Model file for the job. Use its own axes, mm. Face numbers are marked on the shaded views. A direction names the side the tool comes from. Give positions to 0.01 mm unless a question says otherwise; leave off trailing zeros. Order: outer loops, then holes, each group sorted by start corner. A loop starts at its lowest first (then second) coordinate and runs counter-clockwise, first axis right, second up. Notation, with made-up numbers: M 31.25,15 L 70.25,15 A25 cw 70.25,53 Z; hole C -30,37 d9. An arc over 180 degrees is marked long. Return JSON: item names as keys, results as strings. Group by question number.
1. Slice it at D-D on x = 11. List the corners of the cut face in (y, z).
2. Pin check, flat tips, straight feed: pin 1 (1 mm diameter, centred on y = 56, z = 14, fed in from +X); pin 2 (3 mm diameter, centred on x = 23, y = 19, fed in from -Z); pin 3 (2 mm diameter, centred on x = -27, z = 3.5, fed in from +Y); pin 4 (2 mm diameter, centred on y = 41.5, z = 8.5, fed in from +X). Stop position of each tip, or through.
3. 3-axis set-ups, long thin cutter, end or side, ignore diameter. For the marked faces 1, 2 and 3: which of +Z, -Z, +X, -X, +Y, -Y reach the whole face in a straight line?
4. Slice it at C-C on y = 59. List the corners of the cut face in (x, z), then the cut area to 3 significant figures.
5. Wall check: probe 1 along Y at (x, z) = (23.5, 13); probe 2 along X at (y, z) = (59, 13.75); probe 3 along X at (y, z) = (65.5, 12). Give the ranges that are in metal, low to high. Write a range as [from, to].
6. Slice it at A-A on z = 9.15. Give the number of separate pieces and of enclosed holes in the cut face, then the cut area to 3 significant figures.
7. Two-plate mould, pull along X, no slides. Class the marked faces 4, 5 and 6: released by +X, released by -X, zero draft, split by the parting line, or undercut.
from build123d import *

# Parameters (mm, degrees)
SKETCH_W             = 60
SKETCH_H             = 60
PAD_DEPTH            = 4
SKETCH001_R          = 3.5
SKETCH001_R_2        = 1.25
PAD001_DEPTH         = 8
SKETCH009_W          = 5
SKETCH009_H          = 25
POCKET008_DEPTH      = 4
PAD006_DEPTH         = 4
SKETCH015_W          = 22
SKETCH015_H          = 4
PAD007_DEPTH         = 2
SKETCH003_R          = 2.25
PAD008_DEPTH         = 8
SKETCH014_R          = 3.5
SKETCH014_R_2        = 1.25
PAD009_DEPTH         = 15
POCKET_DEPTH         = 4
BODY_PLACEMENT_ANGLE = 180


with BuildPart() as part:
    # Sketch → Pad (new body)
    with BuildSketch(Plane.XY):
        Rectangle(SKETCH_W, SKETCH_H)
    extrude(amount=PAD_DEPTH)

    # Sketch001 (on Face6 of Pad) → Pad001 (join)
    with BuildSketch(Plane.XY.offset(4)):
        with Locations((-17, 17)):
            Circle(SKETCH001_R)
        with Locations((-17, 17)):
            Circle(SKETCH001_R_2, mode=Mode.SUBTRACT)
        with Locations((-17, -17)):
            Circle(SKETCH001_R)
        with Locations((-17, -17)):
            Circle(SKETCH001_R_2, mode=Mode.SUBTRACT)
        with Locations((17, -17)):
            Circle(SKETCH001_R)
        with Locations((17, -17)):
            Circle(SKETCH001_R_2, mode=Mode.SUBTRACT)
        with Locations((17, 17)):
            Circle(SKETCH001_R)
        with Locations((17, 17)):
            Circle(SKETCH001_R_2, mode=Mode.SUBTRACT)
    extrude(amount=PAD001_DEPTH)

    # Sketch009 → Pocket008 (cut)
    with BuildSketch(Plane(origin=(0, 0, 0), x_dir=(1, 0, 0), z_dir=(0, 0, -1))):
        Rectangle(SKETCH009_W, SKETCH009_H)
        with Locations((10, 0)):
            Rectangle(SKETCH009_W, SKETCH009_H)
        with Locations((20, 0)):
            Rectangle(SKETCH009_W, SKETCH009_H)
        with Locations((-10, 0)):
            Rectangle(SKETCH009_W, SKETCH009_H)
        with Locations((-20, 0)):
            Rectangle(SKETCH009_W, SKETCH009_H)
    extrude(amount=-POCKET008_DEPTH, mode=Mode.SUBTRACT)

    # Sketch012 (on Face5 of Pocket008) → Pad006 (join)
    with BuildSketch(Plane.XY.offset(4)):
        Polygon((-30, -12), (-35, -12), (-35, -30), (-33, -28), (-33, -16), (-30, -16), align=None)
    pad006 = extrude(amount=-PAD006_DEPTH)

    # Mirrored005: Pad006 across Sketch012 V_Axis
    add(pad006.mirror(Plane(origin=(0, 0, 4), x_dir=(0, 0, 1), z_dir=(1, 0, 0))))

    # Sketch015 (on Face4 of Pad) → Pad007 (join)
    with BuildSketch(Plane(origin=(-30, 0, 0), x_dir=(0, -1, 0), z_dir=(-1, 0, 0))):
        with Locations((0, 2)):
            Rectangle(SKETCH015_W, SKETCH015_H)
    pad007 = extrude(amount=PAD007_DEPTH)

    # Sketch003 (on Face42 of Pad007) → Pad008 (join)
    with BuildSketch(Plane(origin=(-32, 0, 0), x_dir=(0, -1, 0), z_dir=(-1, 0, 0))):
        with BuildLine():
            ThreePointArc((11, 19), (0, 25.938622), (-11, 19))
            Line((-11, 19), (-11, 0))
            Line((11, 0), (-11, 0))
            Line((11, 19), (11, 0))
        make_face()
        with Locations((0, 13.75)):
            Circle(SKETCH003_R, mode=Mode.SUBTRACT)
    pad008 = extrude(amount=PAD008_DEPTH)

    # Sketch014 → Pad009 (join)
    with BuildSketch(Plane.XY.offset(4)):
        with Locations((-23.5, 23.5)):
            Circle(SKETCH014_R)
        with Locations((-23.5, 23.5)):
            Circle(SKETCH014_R_2, mode=Mode.SUBTRACT)
        with Locations((23.5, 23.5)):
            Circle(SKETCH014_R)
        with Locations((23.5, 23.5)):
            Circle(SKETCH014_R_2, mode=Mode.SUBTRACT)
        with Locations((23.5, -23.5)):
            Circle(SKETCH014_R)
        with Locations((23.5, -23.5)):
            Circle(SKETCH014_R_2, mode=Mode.SUBTRACT)
        with Locations((-23.5, -23.5)):
            Circle(SKETCH014_R)
        with Locations((-23.5, -23.5)):
            Circle(SKETCH014_R_2, mode=Mode.SUBTRACT)
    extrude(amount=PAD009_DEPTH)

    # Sketch016 (on Face58 of Pad009) → Pocket (cut)
    with BuildSketch(Plane.YZ.offset(-32)):
        Polygon((-3.637307, 15.85), (-3.637307, 11.65), (0, 9.55), (3.637307, 11.65), (3.637307, 15.85), (0, 17.95), align=None)
    pocket = extrude(amount=-POCKET_DEPTH, mode=Mode.SUBTRACT)

    # Mirrored: Pad007, Pad008 across YZ
    add(pad007.mirror(Plane.YZ))
    add(pad008.mirror(Plane.YZ))

    # Mirrored006: Pocket across YZ
    add(pocket.mirror(Plane.YZ), mode=Mode.SUBTRACT)


with BuildPart() as part_1:
    # Body placement: moved
    add(part.part.moved(Location((0, 42, 22.9))).rotate(Axis((0, 42, 22.9), (1, 0, 0)), BODY_PLACEMENT_ANGLE))


solid = part_1.part
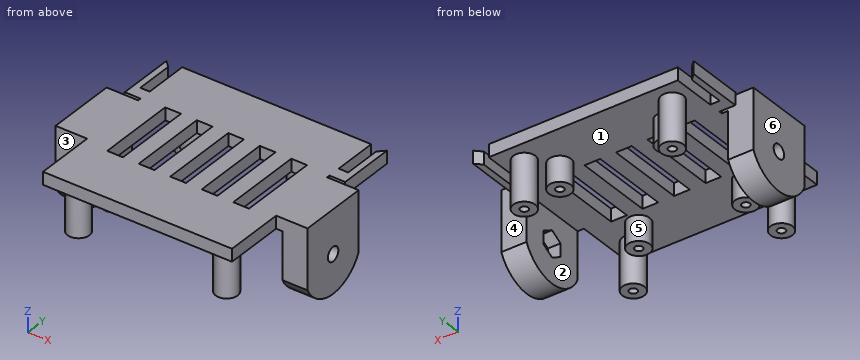
Result:
{
 "1": {"outline": "M 12,18.9 L 29.5,18.9 L 29.5,22.9 L 12,22.9 Z; M 54.5,18.9 L 72,18.9 L 72,22.9 L 54.5,22.9 Z"},
 "2": {"pin 1": "stops at x = 19.45", "pin 2": "stops at z = 3.9", "pin 3": "stops at y = 67.86", "pin 4": "passes through"},
 "3": {"face 1": "-Z", "face 2": "-Z, +Y, -Y", "face 3": "+Z, -Z, -X, -Y"},
 "4": {"outline": "M -35,18.9 L -33,18.9 L -33,22.9 L -35,22.9 Z; M -30,18.9 L -20.5,18.9 L -20.5,10.9 L -18.25,10.9 L -18.25,18.9 L -15.75,18.9 L -15.75,10.9 L -13.5,10.9 L -13.5,18.9 L 13.5,18.9 L 13.5,10.9 L 15.75,10.9 L 15.75,18.9 L 18.25,18.9 L 18.25,10.9 L 20.5,10.9 L 20.5,18.9 L 30,18.9 L 30,22.9 L -30,22.9 Z; M 33,18.9 L 35,18.9 L 35,22.9 L 33,22.9 Z", "area": "328 mm2"},
 "5": {"probe 1": "y = [15, 17.25], [19.75, 22], [62, 64.25], [66.75, 69]", "probe 2": "x = [-20.5, -18.25], [-15.75, -13.5], [13.5, 15.75], [18.25, 20.5]", "probe 3": "x = [-27, -24.75], [-22.25, -20], [20, 22.25], [24.75, 27]"},
 "6": {"separate pieces": "8", "enclosed holes": "4", "area": "392 mm2"},
 "7": {"face 4": "zero draft", "face 5": "undercut", "face 6": "released by -X"}
}
